```python
from build123d import *

# Parameters (mm, degrees)
F1_DEPTH    = 4
F2_R        = 9.99999
F3_R        = 12.5
F6_DEPTH    = 30
F4_R        = 9.3845657054
F7_DEPTH    = 43.1
F8_T1_DEPTH = 50.6060806459
F8_T3_DEPTH = 32.729776757
F8_T5_DEPTH = 33.6001001543
F9_R        = 39
F10_R       = 5


# Not quite as in the source:
# - a fillet or chamfer that OpenCascade refuses, or shapes differently, is made with other operations: its cross-section is extruded or revolved along the edge and cut away or added
# - a fillet or chamfer is up to 0.001 mm smaller than in the source, because OpenCascade refuses the exact size
# - ends of sketch curves that miss each other by under 0.0002 mm in the source are joined


with BuildPart() as f1:
    # F0 (on Front) → F1 (new body)
    with BuildSketch(Plane.XZ):
        Polygon((-70, 0), (0, 0), (64.2787609687, 76.6044443119), (48.9578721063, 89.4601965056), (-4.7950151547, 25.4), (-70, 25.4), align=None)
    extrude(amount=F1_DEPTH)

    # F2 (radius 10 in the source; OpenCascade refuses exactly that, so slightly less here)
    f2_edges = [f1.edges().sort_by_distance(p)[0] for p in [
        (64.278761, -2, 76.604444),
        (48.957872, -2, 89.460197),
    ]]
    fillet(f2_edges, radius=F2_R)

    # F3
    f3_edges = [f1.edges().sort_by_distance(p)[0] for p in [
        (-70, -2, 0),
        (-70, -2, 25.4),
    ]]
    fillet(f3_edges, radius=F3_R)

    # F5 (on face) → F6 (join)
    with BuildSketch(Plane(origin=(0, 0, 0), x_dir=(-1, 0, 0), z_dir=(0, 1, 0))):
        with BuildLine():
            Line((-42.5299960094, 50.6852755372), (-42.5299960094, 81.7997520744))
            ThreePointArc((-42.5299960094, 81.7997520744), (-49.3188826521, 85.3338270849), (-56.618308877, 83.0323268366))
            ThreePointArc((-56.618308877, 83.0323268366), (-60.1523915479, 76.2434337661), (-57.8508912997, 68.9440075412))
            Line((-57.8508912997, 68.9440075412), (-42.5299960094, 50.6852755372))
        make_face()
        Polygon((-6.5299960094, 38.896622741), (-21.5299960094, 56.77292663), (-21.5299960094, 25.6584500928), (-6.5299960094, 7.7821462038), align=None)
    extrude(amount=F6_DEPTH)

    # F4 (on face) → F7 (join)
    with BuildSketch(Plane.XZ.offset(4)):
        with Locations((-57.5, 12.9)):
            Circle(F4_R)
    extrude(amount=-F7_DEPTH)

    # F8: fillet of radius 3 on 6 edges, made by hand

    # F8_s2 → F8_t1 (cut)
    with BuildSketch(Plane.XZ.offset(-50.6060806459)):
        with BuildLine():
            ThreePointArc((16.2318626801, 50.4588572007), (19.5560564394, 51.349572234), (21.5299960094, 48.5304943716))
            Line((21.5299960094, 48.5304943716), (21.5299960094, 56.77292663))
            Line((21.5299960094, 56.77292663), (16.2318626801, 50.4588572007))
        make_face()
        with BuildLine():
            ThreePointArc((11.8281293388, 14.0962156331), (8.5039355794, 13.2055005998), (6.5299960094, 16.0245784622))
            Line((6.5299960094, 16.0245784622), (6.5299960094, 7.7821462038))
            Line((6.5299960094, 7.7821462038), (11.8281293388, 14.0962156331))
        make_face()
        with BuildLine():
            ThreePointArc((47.8281293388, 56.9993449665), (44.5039355794, 56.1086299332), (42.5299960094, 58.9277077956))
            Line((42.5299960094, 58.9277077956), (42.5299960094, 50.6852755372))
            Line((42.5299960094, 50.6852755372), (47.8281293388, 56.9993449665))
        make_face()
    extrude(amount=F8_T1_DEPTH, mode=Mode.SUBTRACT)

    # F8_s4 → F8_t3 (cut)
    with BuildSketch(Plane.XZ.offset(-32.729776757)):
        with BuildLine():
            ThreePointArc((20.8281293388, 24.8219979665), (21.3490738718, 25.7243003656), (21.5299960094, 26.7503607956))
            Line((21.5299960094, 26.7503607956), (21.5299960094, 25.6584500928))
            Line((21.5299960094, 25.6584500928), (20.8281293388, 24.8219979665))
        make_face()
        with BuildLine():
            ThreePointArc((6.5299960094, 37.8047120382), (6.7109181471, 38.8307724682), (7.2318626801, 39.7330748673))
            Line((7.2318626801, 39.7330748673), (6.5299960094, 38.896622741))
            Line((6.5299960094, 38.896622741), (6.5299960094, 37.8047120382))
        make_face()
    extrude(amount=F8_T3_DEPTH, mode=Mode.SUBTRACT)

    # F8_s6 → F8_t5 (cut)
    with BuildSketch(Plane.XZ.offset(-33.6001001543)):
        with BuildLine():
            ThreePointArc((42.5299960094, 80.5949283764), (42.7921129807, 81.8213037352), (43.5326603567, 82.8333765643))
            ThreePointArc((43.5326603567, 82.8333765643), (43.0126982288, 82.3346362508), (42.5299960094, 81.7997520744))
            Line((42.5299960094, 81.7997520744), (42.5299960094, 80.5949283764))
        make_face()
    extrude(amount=F8_T5_DEPTH, mode=Mode.SUBTRACT)

    # F9
    f9_edges = [f1.edges().sort_by_distance(p)[0] for p in [
        (0, -2, 0),
    ]]
    fillet(f9_edges, radius=F9_R)

    # F10
    f10_edges = [f1.edges().sort_by_distance(p)[0] for p in [
        (-4.795015, -2, 25.4),
    ]]
    fillet(f10_edges, radius=F10_R)


solid = f1.part
```
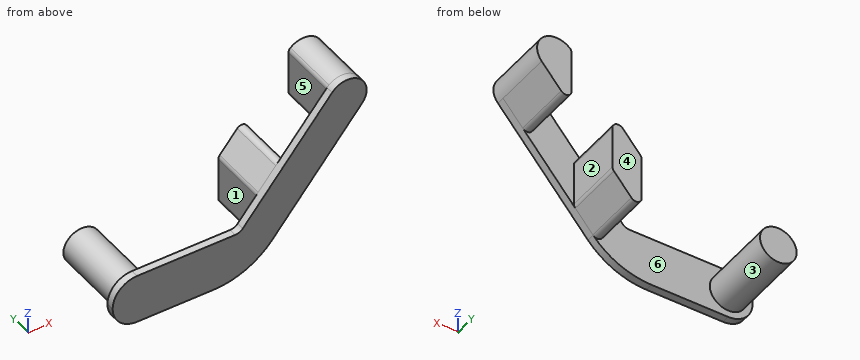
Part model, mm, in its own coordinate system. Face numbers are marked on the shaded views. A direction names the side the tool comes from. Round coordinates to 2 decimals unless told otherwise and drop trailing zeros. Loops run counter-clockwise (first coordinate to the right, second up) from the corner with the lowest first, then second, coordinate; pieces in that order, holes last.
Item 1: Cut at A-A, the plane y = 11.5. Give the cut face in (x, z).
Item 2: Cut at D-D, the plane x = 30. Give the cut face in (y, z), then the cut area to 3 significant figures.
Item 3: Mould opens along X. For the marked faces 4, 5 and 6 say: +X half, -X half, draft (parallel to the pull), parting line (faces both ways), or undercut.
Item 4: Cut at C-C, the plane x = -29.5. Give the cut face in (y, z).
Item 5: Drill centre lines: line 1 (X direction, y = 19, z = 37); line 2 (Y direction, x = 37.5, z = 57); line 3 (X direction, y = 3.5, z = 15). Where is each one in solid material? Low to high.
Item 6: 3-axis set-ups, long thin cutter, end or side, ignore diameter. For the marked faces 1, 2 and 3: which of +Z, -Z, +X, -X, +Y, -Y reach the whole face in a straight line?
Item 7: Cut at B-B, the plane z = 67. Give the cut face in (x, y).
Item 8: Drop flat-ended pins along their axis: P1, Ø9.5, axis at x = 35.5, z = 62.5, coming from the +Y side; P2, Ø4.5, axis at x = -23.5, y = -2, coming from the +Z side; P3, Ø9, axis at x = 50, z = 74.5, coming from the +Y side. Give the stop position or say it passes through.
A:
1. outline: circle Ø18.77 at (-57.5, 12.9); (6.53, 16.02) arc R3 ccw to (11.83, 14.1) - (20.83, 24.82) arc R3 ccw to (21.53, 26.75) - (21.53, 48.53) arc R3 ccw to (16.23, 50.46) - (7.23, 39.73) arc R3 ccw to (6.53, 37.8) - close; (42.53, 58.93) arc R3 ccw to (47.83, 57) - (57.85, 68.94) arc R10 ccw to (56.62, 83.03) arc R10 ccw to (43.53, 82.83) arc R3 ccw to (42.53, 80.59) - close
2. outline: (-4, 35.75) - (0, 35.75) - (0, 66.87) - (-4, 66.87) - close
2. area: 124 mm2
3. face 4: draft
3. face 5: -X half
3. face 6: undercut
4. outline: (-4, 0) - (0, 0) - (0, 25.4) - (-4, 25.4) - close
5. line 1: x = 6.53 to 21.53
5. line 2: y = -4 to 0
5. line 3: x = -66.65 to -48.35, 6.71 to 12.59
6. face 1: +Z, -Z, +Y
6. face 2: +Z, -Z, +X, +Y
6. face 3: +Y
7. outline: (30.11, -4) - (56.22, -4) - (56.22, 30) - (42.53, 30) - (42.53, 0) - (30.11, 0) - close
8. P1: stops at y = 0
8. P2: stops at z = 25.4
8. P3: stops at y = 30
